```python
from build123d import *

# Parameters (mm, degrees)
SKETCH1_W           = 23.83
SKETCH1_H           = 1
BOSS_EXTRUDE1_DEPTH = 21.5
SKETCH2_R           = 1.325
BOSS_EXTRUDE2_DEPTH = 14.25
BOSS_EXTRUDE4_DEPTH = 8
SKETCH5_W           = 21.949336604
SKETCH5_H           = 2.5
BOSS_EXTRUDE5_DEPTH = 45
SKETCH6_R           = 4.25
SKETCH6_R_2         = 1.05
CUT_EXTRUDE1_DEPTH  = 79.646360374
FILLET1_R           = 7
FILLET2_R           = 7
FILLET3_R           = 7
BOSS_EXTRUDE6_START = 41
BOSS_EXTRUDE6_DEPTH = 41


with BuildPart() as part:
    # Sketch1 → Boss-Extrude1 (new body)
    with BuildSketch(Plane(origin=(0, 0, 0), x_dir=(1, 0, 0), z_dir=(0, 1, 0))):
        Rectangle(SKETCH1_W, SKETCH1_H)
    extrude(amount=BOSS_EXTRUDE1_DEPTH)

    # Sketch2 → Boss-Extrude2 (add, symmetric)
    with BuildSketch(Plane(origin=(0, 10.75, 0), x_dir=(1, 0, 0), z_dir=(0, 1, 0))):
        with Locations(Location((-11.915, 0, 0), (0, 0, 270))):
            Circle(SKETCH2_R)
        with Locations(Location((11.915, 0, 0), (0, 0, 270))):
            Circle(SKETCH2_R)
    extrude(amount=BOSS_EXTRUDE2_DEPTH, both=True)

    # Sketch4 → Boss-Extrude4 (add, symmetric)
    with BuildSketch(Plane(origin=(0, 0, 0), x_dir=(0, 0, -1), z_dir=(1, 0, 0))):
        Polygon((-0.5, 17.927447783), (-0.5, 21.5), (-12.5, 33.75), (-35.5, 33.75), (-35.5, 31.25), (-13.550663396, 31.25), align=None)
        Polygon((-0.5, 0), (-0.5, 3.572552217), (-13.550663396, -9.75), (-35.5, -9.75), (-35.5, -12.25), (-12.5, -12.25), align=None)
    extrude(amount=BOSS_EXTRUDE4_DEPTH, both=True)

    # Sketch5 → Boss-Extrude5 (add)
    with BuildSketch(Plane.ZY.offset(8)):
        with Locations((24.525331698, 32.5)):
            Rectangle(SKETCH5_W, SKETCH5_H)
        with Locations((24.525331698, -11)):
            Rectangle(SKETCH5_W, SKETCH5_H)
    extrude(amount=BOSS_EXTRUDE5_DEPTH)

    # Sketch6 → Cut-Extrude1 (cut, through all)
    with BuildSketch(Plane(origin=(0, 33.75, 0), x_dir=(1, 0, 0), z_dir=(0, 1, 0))):
        with Locations(Location((-42.025331698, -24.525331698, 0), (0, 0, 270))):
            Circle(SKETCH6_R)
        with Locations(Location((-49.025331698, -24.525331698, 0), (0, 0, 270))):
            Circle(SKETCH6_R_2)
        with Locations(Location((-42.025331698, -17.525331698, 0), (0, 0, 270))):
            Circle(SKETCH6_R_2)
        with Locations(Location((-35.025331698, -24.525331698, 0), (0, 0, 270))):
            Circle(SKETCH6_R_2)
        with Locations(Location((-42.025331698, -31.525331698, 0), (0, 0, 270))):
            Circle(SKETCH6_R_2)
        with BuildLine():
            ThreePointArc((-53, -24.525331698), (-49.785594076, -16.76506932), (-42.025331698, -13.550663396))
            Line((-42.025331698, -13.550663396), (-53, -13.550663396))
            Line((-53, -13.550663396), (-53, -24.525331698))
        make_face()
        with BuildLine():
            ThreePointArc((-42.025331698, -35.5), (-49.785594076, -32.285594076), (-53, -24.525331698))
            Line((-53, -24.525331698), (-53, -35.5))
            Line((-53, -35.5), (-42.025331698, -35.5))
        make_face()
    extrude(amount=-CUT_EXTRUDE1_DEPTH, mode=Mode.SUBTRACT)

    # Fillet1
    # the kernel refuses this fillet: 7 mm, written as the material it adds along each edge
    with BuildSketch(Plane(origin=(-8, -12.25, 13.550663396), x_dir=(-1, 0, 0), z_dir=(0, 1, 0))) as fillet1_piece_1_section:
        with BuildLine():
            CenterArc((FILLET1_R, -FILLET1_R), FILLET1_R, 90, 90)
            Line((0, -FILLET1_R), (0, 0))
            Line((0, 0), (FILLET1_R, 0))
        make_face()
    fillet1_piece_1 = extrude(amount=2.5, mode=Mode.PRIVATE)
    fillet1_piece_1 = split(fillet1_piece_1, bisect_by=Plane(origin=(-10.015975833, -11.661011889, 11.923032054), z_dir=(0, 0.699779834816443, 0.7143585813751185)), keep=Keep.TOP, mode=Mode.PRIVATE)
    fillet1_piece_1 = split(fillet1_piece_1, bisect_by=Plane(origin=(-10.015975833, -9.911562302, 13.708928508), z_dir=(0, -0.6997798348164429, -0.7143585813751187)), keep=Keep.TOP, mode=Mode.PRIVATE)
    add(fillet1_piece_1)
    with BuildSketch(Plane(origin=(-8, -12.25, 13.550663396), x_dir=(-1, 0, 0), z_dir=(0, 1, 0))) as fillet1_piece_2_section:
        with BuildLine():
            CenterArc((FILLET1_R, -FILLET1_R), FILLET1_R, 90, 90)
            Line((0, -FILLET1_R), (0, 0))
            Line((0, 0), (FILLET1_R, 0))
        make_face()
    fillet1_piece_2 = extrude(amount=20, mode=Mode.PRIVATE)
    fillet1_piece_2 = split(fillet1_piece_2, bisect_by=Plane(origin=(-8.812454151, -9.294822672, 9.605132414), z_dir=(0, 0.699779834816443, 0.7143585813751185)), keep=Keep.TOP, mode=Mode.PRIVATE)
    fillet1_piece_2 = split(fillet1_piece_2, bisect_by=Plane(origin=(-8.812454151, -9.75, 10.768831879), z_dir=(0, 1, 0)), keep=Keep.TOP, mode=Mode.PRIVATE)
    fillet1_piece_2 = split(fillet1_piece_2, bisect_by=Plane(origin=(-8.812454151, -7.545373085, 11.391028867), z_dir=(0, -0.6997798348164429, -0.7143585813751187)), keep=Keep.TOP, mode=Mode.PRIVATE)
    add(fillet1_piece_2)
    with BuildSketch(Plane(origin=(-8, 33.75, 13.550663396), x_dir=(0, 0, -1), z_dir=(0, -1, 0))) as fillet1_piece_3_section:
        with BuildLine():
            CenterArc((FILLET1_R, -FILLET1_R), FILLET1_R, 90, 90)
            Line((0, -FILLET1_R), (0, 0))
            Line((0, 0), (FILLET1_R, 0))
        make_face()
    fillet1_piece_3 = extrude(amount=2.5, mode=Mode.PRIVATE)
    fillet1_piece_3 = split(fillet1_piece_3, bisect_by=Plane(origin=(-10.015975833, 31.411562301, 13.708928507), z_dir=(0, 0.6997798348164431, -0.7143585813751184)), keep=Keep.TOP, mode=Mode.PRIVATE)
    fillet1_piece_3 = split(fillet1_piece_3, bisect_by=Plane(origin=(-10.015975833, 33.161011889, 11.923032054), z_dir=(0, -0.699779834816443, 0.7143585813751185)), keep=Keep.TOP, mode=Mode.PRIVATE)
    add(fillet1_piece_3)
    with BuildSketch(Plane(origin=(-8, 33.75, 13.550663396), x_dir=(0, 0, -1), z_dir=(0, -1, 0))) as fillet1_piece_4_section:
        with BuildLine():
            CenterArc((FILLET1_R, -FILLET1_R), FILLET1_R, 90, 90)
            Line((0, -FILLET1_R), (0, 0))
            Line((0, 0), (FILLET1_R, 0))
        make_face()
    fillet1_piece_4 = extrude(amount=20, mode=Mode.PRIVATE)
    fillet1_piece_4 = split(fillet1_piece_4, bisect_by=Plane(origin=(-8.812454159, 29.045373088, 11.39102887), z_dir=(0, 0.6997798348164431, -0.7143585813751184)), keep=Keep.TOP, mode=Mode.PRIVATE)
    fillet1_piece_4 = split(fillet1_piece_4, bisect_by=Plane(origin=(-8.812454159, 30.794822675, 9.605132416), z_dir=(0, -0.699779834816443, 0.7143585813751185)), keep=Keep.TOP, mode=Mode.PRIVATE)
    fillet1_piece_4 = split(fillet1_piece_4, bisect_by=Plane(origin=(-8.812454159, 31.25, 10.768831882), z_dir=(0, -1, 0)), keep=Keep.TOP, mode=Mode.PRIVATE)
    add(fillet1_piece_4)
    # the kernel refuses this fillet: 7 mm, written as the material it takes off along each edge
    with BuildSketch(Plane(origin=(8, 7.75, 35.5), x_dir=(0, 0, -1), z_dir=(0, -1, 0))) as fillet1_2_piece_1:
        with BuildLine():
            CenterArc((FILLET1_R, -FILLET1_R), FILLET1_R, 90, 90)
            Line((0, -FILLET1_R), (0, 0))
            Line((0, 0), (FILLET1_R, 0))
        make_face()
    extrude(amount=37.5, mode=Mode.SUBTRACT)
    with BuildSketch(Plane(origin=(8, 51.25, 35.5), x_dir=(-1, 0, 0), z_dir=(0, -1, 0))) as fillet1_2_piece_2:
        with BuildLine():
            CenterArc((FILLET1_R, FILLET1_R), FILLET1_R, 180, 90)
            Line((0, FILLET1_R), (0, 0))
            Line((0, 0), (FILLET1_R, 0))
        make_face()
    extrude(amount=37.5, mode=Mode.SUBTRACT)

    # Fillet2
    fillet2_edges = [part.edges().sort_by_distance(p)[0] for p in [
        (0, 17.927447783, 0.5),
        (0, 3.572552217, 0.5),
    ]]
    fillet(fillet2_edges, radius=FILLET2_R)

    # Fillet3
    # the kernel refuses this fillet: 7 mm, written as the material it adds along each edge
    with BuildSketch(Plane(origin=(-8, 21.5, 0.5), x_dir=(0, 0.7143585813744706, 0.6997798348171044), z_dir=(1, 0, 0))) as fillet3_piece_1:
        with BuildLine():
            CenterArc((2.380920079, -7), FILLET3_R, 90, 26.110260914)
            Line((-0.699779835, -0.714358581), (0, 0))
            Line((0, 0), (2.380920079, 0))
        make_face()
    extrude(amount=16)
    with BuildSketch(Plane(origin=(8, 0, 0.5), x_dir=(0, 0, -1), z_dir=(-1, 0, 0))) as fillet3_piece_2:
        with BuildLine():
            CenterArc((3.33439021, 6.599289533), FILLET3_R, 224.409342785, 26.110260914)
            Line((-1.666119859, 1.70083069), (0, 0))
            Line((0, 0), (1, 0))
        make_face()
    extrude(amount=16)

    # Sketch8 → Boss-Extrude6 (add)
    with BuildSketch(Plane(origin=(0, -9.75, 0), x_dir=(1, 0, 0), z_dir=(0, 1, 0)).offset(BOSS_EXTRUDE6_START)):
        with BuildLine():
            ThreePointArc((1, -35.5), (5.949747468, -33.449747468), (8, -28.5))
            Line((8, -28.5), (5, -28.5))
            ThreePointArc((5, -28.5), (3.422054899, -30.922054899), (1, -32.5))
            Line((1, -32.5), (1, -35.5))
        make_face()
    extrude(amount=-BOSS_EXTRUDE6_DEPTH)


solid = part.part
```
Source: CAD feature listing. Evaluate the final solid. Frame: model axes, mm. A direction names the side the tool comes from. Give positions to 0.01 mm unless a question says otherwise; leave off trailing zeros. Order: outer loops, then holes, each group sorted by start corner. A loop starts at its lowest first (then second) coordinate and runs counter-clockwise, first axis right, second up. Notation, with made-up numbers: (59, 5) -> (108, 5) arc R25 ccw to (108, 39) -> close; hole circle Ø3 at (-27.75, 14). An arc over 180 degrees is marked (long way). Use a Markdown table: item, result.
Q1. Section C-C (z = 8). Return the cut outline in (x, y), and give its area (3 significant figures).
A:
| item | result |
|---|---|
| outline | (-8.15, -7.66) -> (8, -7.66) -> (8, -4.08) -> (-8.15, -4.08) -> close; (-8.15, 25.58) -> (8, 25.58) -> (8, 29.16) -> (-8.15, 29.16) -> close |
| area | 115 mm^2 |
Q2. Section D-D (x = -39.5). Return the cut outline in (y, z).
A:
| item | result |
|---|---|
| outline | (-12.25, 13.55) -> (-9.75, 13.55) -> (-9.75, 21.11) -> (-12.25, 21.11) -> close; (-12.25, 27.94) -> (-9.75, 27.94) -> (-9.75, 35.5) -> (-12.25, 35.5) -> close; (31.25, 13.55) -> (33.75, 13.55) -> (33.75, 21.11) -> (31.25, 21.11) -> close; (31.25, 27.94) -> (33.75, 27.94) -> (33.75, 35.5) -> (31.25, 35.5) -> close |
Q3. Section B-B (x = -23). Return the cut outline in (y, z), and give its area (3 significant figures).
A:
| item | result |
|---|---|
| outline | (-12.25, 13.55) -> (-9.75, 13.55) -> (-9.75, 35.5) -> (-12.25, 35.5) -> close; (31.25, 13.55) -> (33.75, 13.55) -> (33.75, 35.5) -> (31.25, 35.5) -> close |
| area | 110 mm^2 |
Q4. Material intervals for line 1 (Y direction, x = -23, z = 28); line 2 (X direction, y = -0.5, z = 1); line 3 (Z direction, x = 2, y = 15), sorted ascending. Write a range as [from, to].
A:
| item | result |
|---|---|
| line 1 | [-12.25, -9.75], [31.25, 33.75] |
| line 2 | [-12.78, -11.05], [-8, 8], [11.05, 12.78] |
| line 3 | [-0.5, 0.5], [32.02, 35.43] |
Q5. Pull-direction query (Y, two-part tool) for faces 1 (the face through (1, 11, 34)), 2 (the face through (-50.05, -10.98, 24.3)), 3 (the face through (0.355, -7.049, 7.405)), 4 (the face through (0, 11, 0.5)); classes: +Y half, -Y half, draft (parallel to the pull), parting line (faces both ways), or undercut.
A:
| item | result |
|---|---|
| face 1 | undercut |
| face 2 | draft |
| face 3 | -Y half |
| face 4 | undercut |
Q6. Section A-A (y = 14). Return the cut outline in (x, z) (3 decimals), and give its area (3 significant figures).
A:
| item | result |
|---|---|
| outline | (-10.688, -0.5) -> (10.688, -0.5) arc R1.325 ccw (long way) to (10.688, 0.5) -> (-10.688, 0.5) arc R1.325 ccw (long way) to start; (1, 32.5) arc R7 cw to (5, 28.5) -> (8, 28.5) arc R7 ccw to (1, 35.5) -> close |
| area | 60.5 mm^2 |
Q7. Access query for faces 5 (the face through (0.112, 3.82, 1.005)), 6 (the face through (12, 25, 0)), 7 (the face through (-28, -11, 13.551)). Directions: +Z, -Z, +X, -X, +Y, -Y. A direction counts if a zero-diameter tool reaches every point of the face in a straight line with its end or side. Return the directions, or none.
A:
| item | result |
|---|---|
| face 5 | none |
| face 6 | +Z, -Z, +X, -X, +Y |
| face 7 | -Z, -X, +Y, -Y |
Q8. First-contact query: P1, Ø5, axis at x = -4, y = 19, coming from the -Z side; P2, Ø1.1, axis at x = -9.5, z = 0, coming from the -Y side; P3, Ø3, axis at y = -1, z = 4, coming from the +X side. Flat tips, straight axial feed; report the tip coordinate or a pass-through.
A:
| item | result |
|---|---|
| P1 | z = -0.5 |
| P2 | y = 0 |
| P3 | x = 8 |
